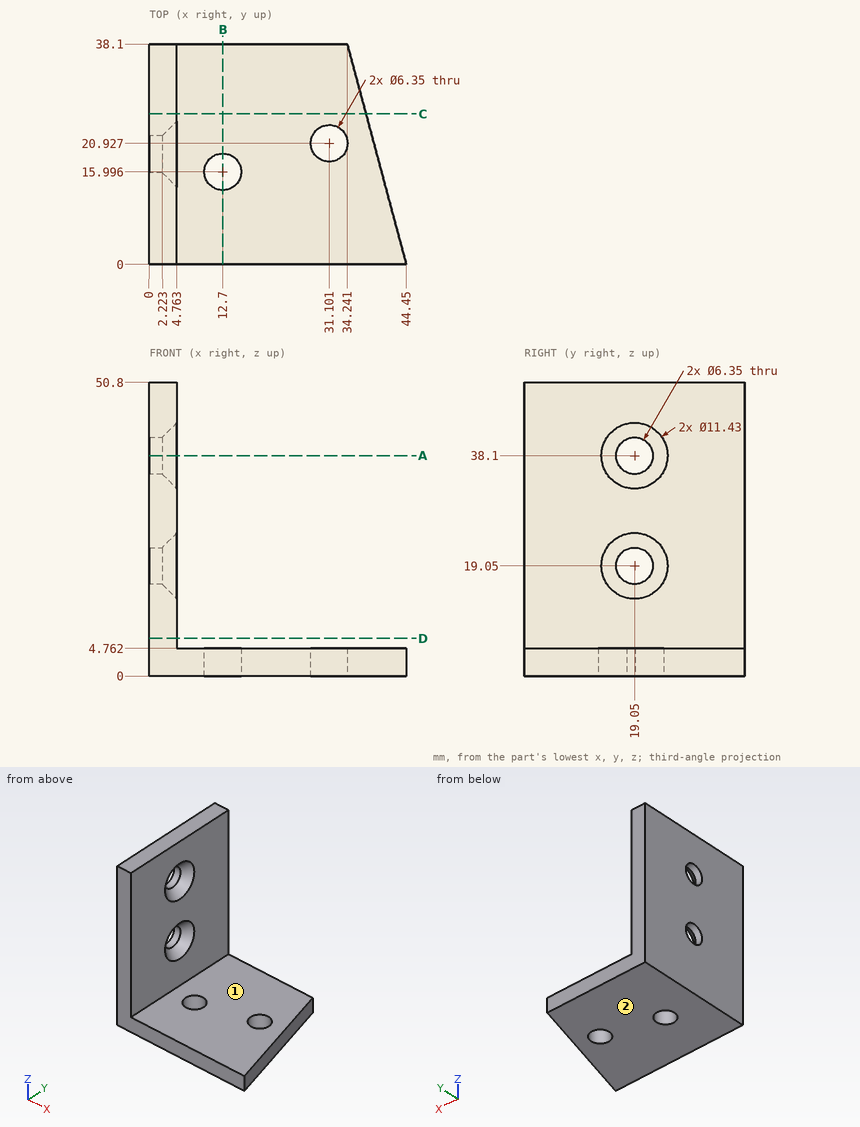
Print and shaded views of the part. All mm, measured from the part's lowest x, y and z. A direction names the side the tool comes from. Coordinates: 2 decimals unless noted, no trailing zeros. Loops run counter-clockwise (first coordinate to the right, second up) from the corner with the lowest first, then second, coordinate; pieces in that order, holes last. Notation, with made-up numbers: (35, 69.5) -> (58, 69.5) arc R31 cw to (58, 102.5) -> close; hole circle Ø5 at (62.25, 2.25). An arc over 180 degrees is marked (long way). Use one line per item in the form item = value. Start each with the question number.
(1) Probe probe 1 along Y at (x, z) = (12.7, 2.15); probe 2 along Z at (x, y) = (4, 23) (1 decimal); probe 3 along Y at (x, z) = (1.1, 19.05) (1 decimal). List the from-to ranges inside material, lowest first. Write a range as from..to.
(2) Tool access for the marked faces 1 and 2: list every direction of +Z, -Z, +X, -X, +Y, -Y with a clear straight run to the whole face (end or side of a thin tool).
(3) Cut at B-B on x = 12.7. Give the cut face in (y, z), and give its area (3 significant figures).
(4) Cut at A-A on z = 38.1. Give the cut face in (x, y) (1 decimal), and give its area (3 significant figures).
(5) Cut at D-D on z = 6.5. Give the cut face in (x, y).
(6) Flat gauge pins, fed straight in: pin 1 (6 mm diameter, centred on x = 20, y = 5.5, fed in from +Z); pin 2 (8.5 mm diameter, centred on y = 19.05, z = 38.1, fed in from +X); pin 3 (10 mm diameter, centred on y = 19.05, z = 19.05, fed in from +X); pin 4 (5.5 mm diameter, centred on x = 12.7, y = 16, fed in from +Z). Where does each tip first touch, or does it go through?
(7) Cut at C-C on y = 26. Give the cut face in (x, z).
Values:
q1.probe_1 = 0..12.82, 19.17..38.1
q1.probe_2 = 0..16.1, 22..35.1, 41.1..50.8
q1.probe_3 = 0..15.9, 22.2..38.1
q2.face_1 = +Z, +X, +Y, -Y
q2.face_2 = -Z, +X, -X, +Y, -Y
q3.outline = (0, 0) -> (12.82, 0) -> (12.82, 4.76) -> (0, 4.76) -> close; (19.17, 0) -> (38.1, 0) -> (38.1, 4.76) -> (19.17, 4.76) -> close
q3.area = 151 mm2
q4.outline = (0, 0) -> (4.8, 0) -> (4.8, 13.3) -> (2.2, 15.9) -> (0, 15.9) -> close; (0, 22.2) -> (2.2, 22.2) -> (4.8, 24.8) -> (4.8, 38.1) -> (0, 38.1) -> close
q4.area = 145 mm2
q5.outline = (0, 0) -> (4.76, 0) -> (4.76, 38.1) -> (0, 38.1) -> close
q6.pin_1 = 4.76
q6.pin_2 = 3.3
q6.pin_3 = 4.05
q6.pin_4 = through
q7.outline = (0, 0) -> (37.48, 0) -> (37.48, 4.76) -> (4.76, 4.76) -> (4.76, 50.8) -> (0, 50.8) -> close
